Autodesk Inventor part; units mm, degrees
ref_plane "YZ Plane" through (0, 0, 0) normal (1, 0, 0) x (0, 1, 0)
ref_plane "XZ Plane" through (0, 0, 0) normal (0, 1, 0) x (-1, 0, 0)
ref_plane "XY Plane" through (0, 0, 0) normal (0, 0, 1) x (1, 0, 0)
sketch "Sketch1" plane through (0, 0, 0) normal (0, 1, 0) x (-1, 0, 0)
  arc A0 (0, 42.545) -> (0, -42.545) centre (0, 0) ccw
  arc A1 (0, 40.005) -> (0, -40.005) centre (0, 0) ccw
  line L0 (0, 42.545) -> (0, 40.005)
  line L1 (0, -40.005) -> (0, -42.545)
  line L2 (-40.005, 0) -> (-42.545, 0)
  line L3 (-42.545, 0) -> (-42.545, -25.4)
  line L4 (-42.545, -25.4) -> (-34.1309, -25.4)
  line L5 (-40.005, 0) -> (-42.545, 0)
  line L6 (-42.545, 0) -> (-42.545, 25.4)
  line L7 (-42.545, 25.4) -> (-34.1309, 25.4)
  dimension "d0" = 85.09
  dimension "d1" = 80.01
  dimension "d2" = 25.4
  dimension "d3" = 25.4
extrude "Extrusion1" add sketch "Sketch1" along normal blind 101.6
properties part number "BlockSlideTestTube"
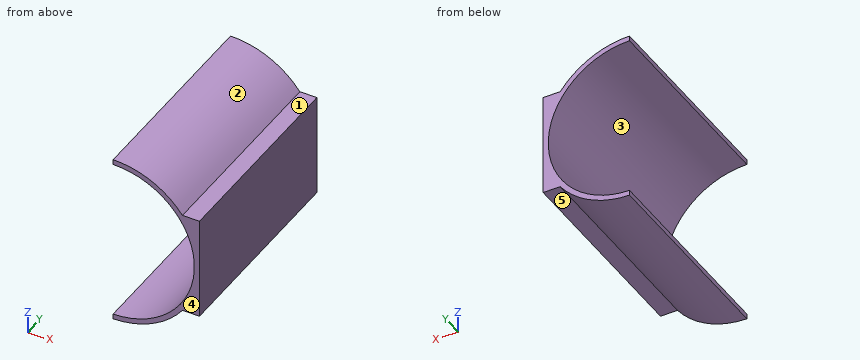
The listing builds one solid part. Answer for the finished solid, in the listing's coordinates (mm). Face numbers are marked on the shaded views. A direction names the side the tool comes from. Coordinates: 2 decimals unless noted, no trailing zeros. Loops run counter-clockwise (first coordinate to the right, second up) from the corner with the lowest first, then second, coordinate; pieces in that order, holes last. Notation, with made-up numbers: M -35.5,62.25 L -21.5,62.25 A31 cw -21.5,97.25 Z; hole C 23,35.5 d11. An arc over 180 degrees is marked long. Answer in a Markdown table with one row per item.
1) Which of the six approach directions +Z, -Z, +X, -X, +Y, -Y give full straight-line access (tool end or side, diameter ignored) to the marked faces 4 and 5?
Answers below:
| item | result |
|---|---|
| face 4 | +Z, -Z, +X, -X, -Y |
| face 5 | -Z, +X, +Y, -Y |
2) Determine the mould class of the marked faces 1, 2 and 3 for opening direction X: released by +X, released by -X, zero draft, split by the parting line, or undercut.
Answers below:
| item | result |
|---|---|
| face 1 | zero draft |
| face 2 | released by +X |
| face 3 | released by -X |
3) Find the intervals of material crossed by probe 1 along Z at (x, y) = (15.5, 69); probe 2 along Z at (x, y) = (37, 17); probe 3 along X at (y, z) = (19.5, -29), in increasing order.
Answers below:
| item | result |
|---|---|
| probe 1 | -39.62 to -36.88, 36.88 to 39.62 |
| probe 2 | -25.4 to -15.21, 15.21 to 25.4 |
| probe 3 | 27.56 to 31.13 |
4) Find section D-D (x = 28). Determine the outline of the cut face in (y, z).
Answers below:
| item | result |
|---|---|
| outline | M 0,-32.03 L 101.6,-32.03 L 101.6,-28.57 L 0,-28.57 Z; M 0,28.57 L 101.6,28.57 L 101.6,32.03 L 0,32.03 Z |
5) Given pin 1 (4 mm diameter, centred on x = 38, y = 76, fed in from -Z); pin 2 (1.5 mm diameter, centred on x = 9, y = 81, fed in from -Z); pin 3 (5 mm diameter, centred on x = 22, y = 23.5, fed in from -Z); pin 4 (10 mm diameter, centred on x = 33, z = -5.5, fed in from +Y), each flat-ended and moving along its own axis, determine where each tip first touches the part or whether it passes through.
Answers below:
| item | result |
|---|---|
| pin 1 | z = -25.4 |
| pin 2 | z = -41.74 |
| pin 3 | z = -37.81 |
| pin 4 | through |
6) Find section B-B (z = 0). Determine the outline of the cut face in (x, y) (3 decimals).
Answers below:
| item | result |
|---|---|
| outline | M 40.005,0 L 42.545,0 L 42.545,101.6 L 40.005,101.6 Z |
7) Find section A-A (x = 20.5). Determine the outline of the cut face in (y, z), then the cut area to 3 significant figures.
Answers below:
| item | result |
|---|---|
| outline | M 0,-37.28 L 101.6,-37.28 L 101.6,-34.35 L 0,-34.35 Z; M 0,34.35 L 101.6,34.35 L 101.6,37.28 L 0,37.28 Z |
| area | 595 mm^2 |
8) Find section C-C (y = 45.5). Determine the outline of the cut face in (x, z) (3 decimals).
Answers below:
| item | result |
|---|---|
| outline | M 0,-42.545 A42.545 ccw 34.131,-25.4 L 42.545,-25.4 L 42.545,25.4 L 34.131,25.4 A42.545 ccw 0,42.545 L 0,40.005 A40.005 cw 0,-40.005 Z |
